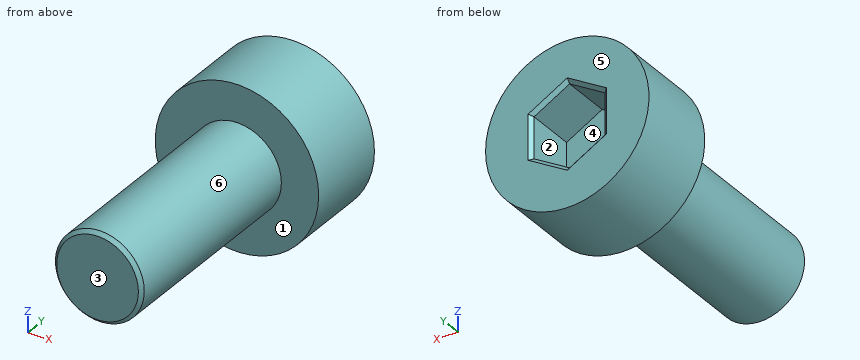
```python
from build123d import *

# Parameters (mm, degrees)
SKETCH_1_R          = 2.3
EXTRUDE_1_DEPTH     = 2.4
CUT_EXTRUDE_1_DEPTH = 1.5
SKETCH_3_R          = 1.25
EXTRUDE_2_DEPTH     = 6
CHAMFER_1_SIZE      = 0.1


with BuildPart() as part:
    # 草图1 → 凸台-拉伸1 (new body)
    with BuildSketch(Plane(origin=(0, 0, 0), x_dir=(1, 0, 0), z_dir=(0, 1, 0))):
        Circle(SKETCH_1_R)
    extrude(amount=EXTRUDE_1_DEPTH)

    # 草图2 → 切除-拉伸1 (cut)
    with BuildSketch(Plane(origin=(0, 2.4, 0), x_dir=(1, 0, 0), z_dir=(0, 1, 0))):
        Polygon((0, -1.154700538), (1, -0.577350269), (1, 0.577350269), (0, 1.154700538), (-1, 0.577350269), (-1, -0.577350269), align=None)
    extrude(amount=-CUT_EXTRUDE_1_DEPTH, mode=Mode.SUBTRACT)

    # 草图3 → 凸台-拉伸2 (add)
    with BuildSketch(Plane.XZ):
        Circle(SKETCH_3_R)
    extrude(amount=EXTRUDE_2_DEPTH)

    # 倒角1
    chamfer_1_edges = [part.edges().sort_by_distance(p)[0] for p in [
        (-0.5, 2.4, 0.866025404),
        (0.5, 2.4, 0.866025404),
        (1, 2.4, 0),
        (0.5, 2.4, -0.866025404),
        (-0.5, 2.4, -0.866025404),
        (-1, 2.4, 0),
        (-1.25, -6, 0),
    ]]
    chamfer(chamfer_1_edges, length=CHAMFER_1_SIZE)


solid = part.part
```
Can you work these out from the model? Positions are in its coordinate system, mm. Face numbers are marked on the shaded views. A direction names the side the tool comes from. Give positions to 0.01 mm unless a question says otherwise; leave off trailing zeros. Loops run counter-clockwise (first coordinate to the right, second up) from the corner with the lowest first, then second, coordinate; pieces in that order, holes last. Notation, with made-up numbers: M -10,20.5 L 32,20.5 A19 ccw 32,27.5 Z; hole C 15.5,60.5 d9. An arc over 180 degrees is marked long. Use one line per item in the form item = value. Start each with the question number.
(1) I'm going to push flat-ended pins straight in: P1, Ø2, axis at x = 0.5, z = -0.5, coming from the +Y side; P2, Ø1.5, axis at y = -1, z = -1, coming from the +X side; P3, Ø1.5, axis at y = 0.5, z = -1.5, coming from the -X side. Where does each tip first touch, or does it pass through?
(2) I want a section at B-B, the plane z = 0. Write out the boundary of the cut face in (x, y), and give its area (3 significant figures).
(3) I want a section at C-C, the plane y = -4.5. Write out the boundary of the cut face in (x, z), and give its area (3 significant figures).
(4) I want a section at D-D, the plane x = 1.9. Write out the boundary of the cut face in (y, z).
(5) On a 3-axis mill with a long thin cutter (end or side, diameter ignored), from which of +Z, -Z, +X, -X, +Y, -Y can I reach the whole of each face in a straight line? I mean the marked faces 1, 2 and 3. Say none if no direction works.
(6) Thinking about a two-plate mould opening in X: for the marked faces 4, 5 and 6, which applies, released by +X, released by -X, zero draft, split by the parting line, or undercut?
(7) I want a section at A-A, the plane y = 1.5. Write out the boundary of the cut face in (x, z), and give its area (3 significant figures).
(8) Please list where these lines run through material, in increasing order: line 1 (Y direction, x = -0.2, z = 0.6); line 2 (Y direction, x = 2, z = 0.05); line 3 (X direction, y = 1.25, z = -0.1).
Worked out:
q1.P1 = 2.4
q1.P2 = 1.22
q1.P3 = -2.17
q2.outline = M -2.3,0 L -1.25,0 L -1.25,-5.9 L -1.15,-6 L 1.15,-6 L 1.25,-5.9 L 1.25,0 L 2.3,0 L 2.3,2.4 L 1.1,2.4 L 1,2.3 L 1,0.9 L -1,0.9 L -1,2.3 L -1.1,2.4 L -2.3,2.4 Z
q2.area = 23.0 mm²
q3.outline = C 0,0 d2.5
q3.area = 4.91 mm²
q4.outline = M 0,-1.3 L 2.4,-1.3 L 2.4,1.3 L 0,1.3 Z
q5.face_1 = -Y
q5.face_2 = +Y
q5.face_3 = +Z, -Z, +X, -X, -Y
q6.face_4 = undercut
q6.face_5 = zero draft
q6.face_6 = split by the parting line
q7.outline = C 0,0 d4.6; hole M -1,-0.58 L 0,-1.15 L 1,-0.58 L 1,0.58 L 0,1.15 L -1,0.58 Z
q7.area = 13.2 mm²
q8.line_1 = -6 to 0.9
q8.line_2 = 0 to 2.4
q8.line_3 = -2.3 to -1, 1 to 2.3
